Geometry: final body of the model. Coordinates: model frame, mm. Face numbers are marked on the shaded views. A direction names the side the tool comes from. Give positions to 0.01 mm unless a question says otherwise; leave off trailing zeros. Loops run counter-clockwise (first coordinate to the right, second up) from the corner with the lowest first, then second, coordinate; pieces in that order, holes last. Notation, with made-up numbers: (80, -20.75) - (102, -20.75) arc R19 cw to (102, 11.25) - close; hole circle Ø11 at (24, 4.5). An arc over 180 degrees is marked (long way). Use CSV: the item, a comma, the result in double quotes. Start each with the question number.
```python
from build123d import *

# Parameters (mm, degrees)
F0_R     = 50
F1_DEPTH = 40
F2_R     = 42.978315
F3_DEPTH = 100
F4_R     = 19.003957
F5_DEPTH = 50
F6_R     = 5.601442
F7_DEPTH = 30


with BuildPart() as f1:
    # F0 (on Front) → F1 (new body)
    with BuildSketch(Plane.XZ):
        Circle(F0_R)
    extrude(amount=F1_DEPTH)

    # F2 (on Front) → F3 (join)
    with BuildSketch(Plane.XZ):
        Circle(F2_R)
    extrude(amount=F3_DEPTH)

    # F4 (on face) → F5 (join)
    with BuildSketch(Plane.XZ.offset(100)):
        Circle(F4_R)
    extrude(amount=F5_DEPTH)

    # F6 (on face) → F7 (join)
    with BuildSketch(Plane.XZ.offset(150)):
        Circle(F6_R)
    extrude(amount=F7_DEPTH)


solid = f1.part
```
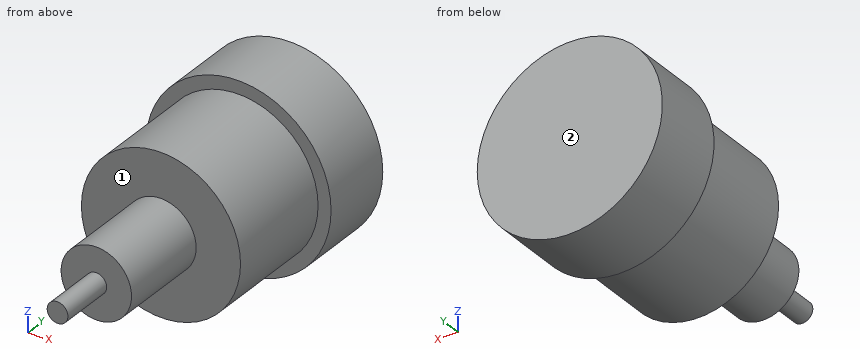
Item 1: Ray query, probe 1 along Y at (x, z) = (39.5, -28.5); probe 2 along Y at (x, z) = (-2, -27.5); probe 3 along X at (y, z) = (-17.5, -43). Return the intervals inside material, ascending.
Item 2: Section D-D (z = 11.5). Output: boundary loops of the cut face in (x, y).
Item 3: Pin query (flat end, axial travel): pin 1 Ø1 at (y, z) = (-68.5, -11) entering from -X; pin 2 Ø1 at (x, y) = (18, -123) entering from -Z; pin 3 Ø3 at (x, y) = (-8, -74) entering from -Z. Return the tip coordinate at first contact, or that it passes through.
Item 4: Section C-C (y = -52). Output: boundary loops of the cut face in (x, z), plus the area to 3 significant figures.
Item 5: Section A-A (z = 0). Output: boundary loops of the cut face in (x, y), plus the area to 3 significant figures.
Item 6: Reachability of the marked faces 1 and 2 from +Z, -Z, +X, -X, +Y, -Y: full face, straight path, thin tool, end or side. Return the list, or none.
Item 7: Section B-B (x = 0). Output: boundary loops of the cut face in (y, z), plus the area to 3 significant figures.
Outcome:
1,probe 1,"y = -40 to 0"
1,probe 2,"y = -100 to 0"
1,probe 3,"x = -25.51 to 25.51"
2,outline,"(-48.66, -40) - (-41.41, -40) - (-41.41, -100) - (-15.13, -100) - (-15.13, -150) - (15.13, -150) - (15.13, -100) - (41.41, -100) - (41.41, -40) - (48.66, -40) - (48.66, 0) - (-48.66, 0) - close"
3,pin 1,"stops at x = -41.68"
3,pin 2,"stops at z = -7.41"
3,pin 3,"stops at z = -42.48"
4,outline,"circle Ø85.96 at (0, 0)"
4,area,"5,800 mm2"
5,outline,"(-50, -40) - (-42.98, -40) - (-42.98, -100) - (-19, -100) - (-19, -150) - (-5.6, -150) - (-5.6, -180) - (5.6, -180) - (5.6, -150) - (19, -150) - (19, -100) - (42.98, -100) - (42.98, -40) - (50, -40) - (50, 0) - (-50, 0) - close"
5,area,"11,400 mm2"
6,face 1,"-Y"
6,face 2,"+Z, -Z, +X, -X, +Y"
7,outline,"(-180, -5.6) - (-150, -5.6) - (-150, -19) - (-100, -19) - (-100, -42.98) - (-40, -42.98) - (-40, -50) - (0, -50) - (0, 50) - (-40, 50) - (-40, 42.98) - (-100, 42.98) - (-100, 19) - (-150, 19) - (-150, 5.6) - (-180, 5.6) - close"
7,area,"11,400 mm2"
